Here's the drawing with two shaded views (mm, measured from the low corner). I have some questions. Give positions to 0.01 mm unless a question says otherwise; leave off trailing zeros. Loops run counter-clockwise (first coordinate to the right, second up) from the corner with the lowest first, then second, coordinate; pieces in that order, holes last. Notation, with made-up numbers: M -13,1 L 19,1 A31 cw 19,40 Z; hole C -15,-27.75 d2. An arc over 180 degrees is marked long. Use a Markdown table: item, result. Add a question column.
1) We'd pull the mould along X, two halves only. Please class the marked faces 1, 2 and 3: +X half, -X half, draft (parallel to the pull), parting line (faces both ways), or undercut.
2) If I drill on line 1 along Z through (x, y) = (53.57, 2.25); line 2 along X through (y, z) = (8.15, 30), over which ranges is the centre line in solid material (lowest first)? Write a range as [from, to].
3) Suppose I cut it at A-A on z = 6.43. List the corners of the cut face in (x, y) for me (3 decimals), and give its area (3 significant figures).
4) Will these pins go through, and if not, where does the flat tip stop? pin 1 Ø3 at (x, z) = (6.43, 53.57) entering from +Y; pin 2 Ø13 at (x, z) = (30, 30) entering from +Y.
5) Suppose I cut it at C-C on z = 30. List the corners of the cut face in (x, y) for me (3 decimals).
6) Suppose I cut it at D-D on x = 30. List the corners of the cut face in (y, z) for me (3 decimals), and give its area (3 significant figures).
7) Suppose I cut it at B-B on x = 53.57. List the corners of the cut face in (y, z) for me (3 decimals).
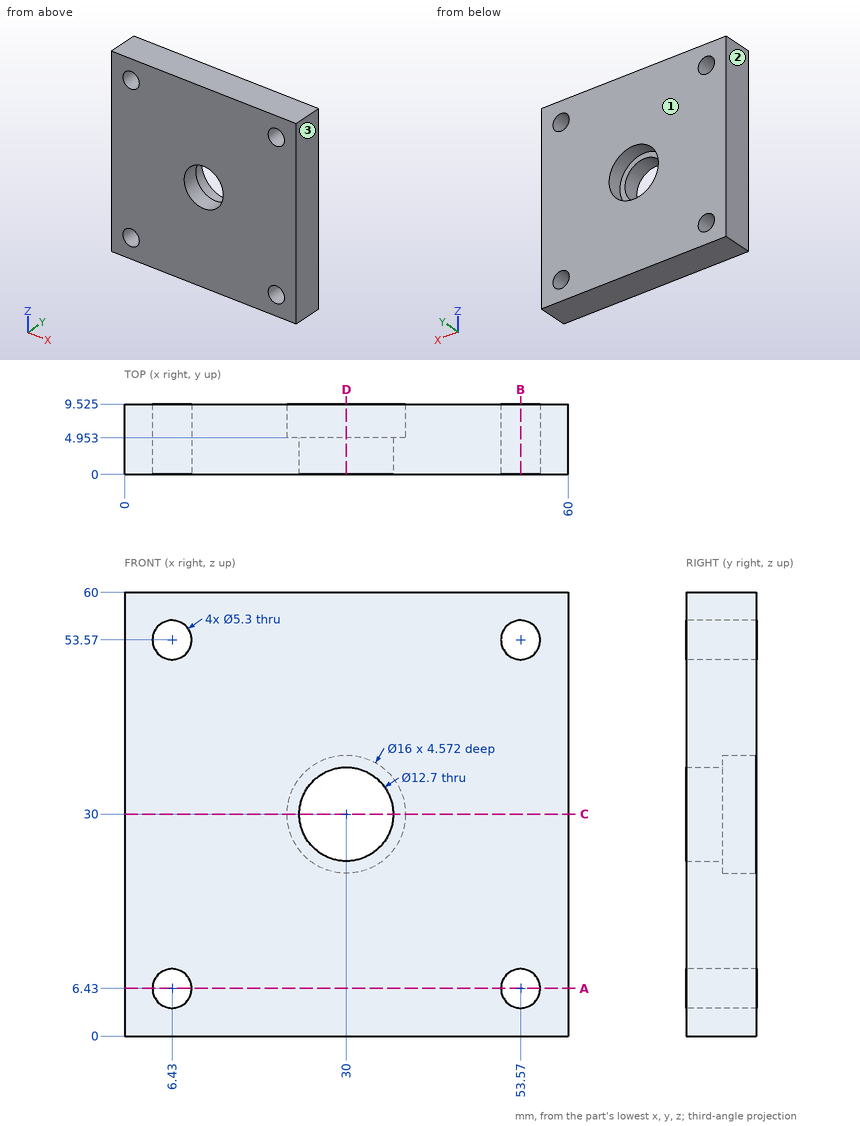
Answer block:
| question | item | result |
|---|---|---|
| 1 | face 1 | draft |
| 1 | face 2 | -X half |
| 1 | face 3 | +X half |
| 2 | line 1 | z = [0, 3.78], [9.08, 50.92], [56.22, 60] |
| 2 | line 2 | x = [0, 22], [38, 60] |
| 3 | outline | M 0,0 L 3.78,0 L 3.78,9.525 L 0,9.525 Z; M 9.08,0 L 50.92,0 L 50.92,9.525 L 9.08,9.525 Z; M 56.22,0 L 60,0 L 60,9.525 L 56.22,9.525 Z |
| 3 | area | 471 mm^2 |
| 4 | pin 1 | passes through |
| 4 | pin 2 | stops at y = 4.95 |
| 5 | outline | M 0,0 L 23.65,0 L 23.65,4.953 L 22,4.953 L 22,9.525 L 0,9.525 Z; M 36.35,0 L 60,0 L 60,9.525 L 38,9.525 L 38,4.953 L 36.35,4.953 Z |
| 6 | outline | M 0,0 L 9.525,0 L 9.525,22 L 4.953,22 L 4.953,23.65 L 0,23.65 Z; M 0,36.35 L 4.953,36.35 L 4.953,38 L 9.525,38 L 9.525,60 L 0,60 Z |
| 6 | area | 435 mm^2 |
| 7 | outline | M 0,0 L 9.525,0 L 9.525,3.78 L 0,3.78 Z; M 0,9.08 L 9.525,9.08 L 9.525,50.92 L 0,50.92 Z; M 0,56.22 L 9.525,56.22 L 9.525,60 L 0,60 Z |
